Verification items for the finished model (mm, model axes). Give positions to 0.01 mm unless a question says otherwise; leave off trailing zeros. Loops run counter-clockwise (first coordinate to the right, second up) from the corner with the lowest first, then second, coordinate; pieces in that order, holes last. Notation, with made-up numbers: M 70.5,87.5 L 106.5,87.5 A32 cw 106.5,118.5 Z; hole C -1.5,53.5 d11. An arc over 180 degrees is marked long. Use CSV: the item, a comma, the result in double quotes.
from build123d import *

# Parameters (mm, degrees)
IZIM1_R                     = 3
Y_KSEKLIK_EKSTR_ZYON6_DEPTH = 99
IZIM2_R                     = 2
Y_KSEKLIK_EKSTR_ZYON7_DEPTH = 4
RADYUS1_SIZE                = 0.5
Y_KSEKLIK_EKSTR_ZYON8_START = 4
IZIM5_R                     = 2
Y_KSEKLIK_EKSTR_ZYON8_DEPTH = 4
RADYUS2_SIZE                = 0.5


with BuildPart() as part:
    # Çizim1 → Yükseklik-Ekstrüzyon6 (new, symmetric)
    with BuildSketch(Plane(origin=(0, 0, 0), x_dir=(1, 0, 0), z_dir=(0, 1, 0))):
        with Locations(Location((0, 0, 0), (0, 0, 270))):
            Circle(IZIM1_R)
    extrude(amount=Y_KSEKLIK_EKSTR_ZYON6_DEPTH, both=True)

    # Çizim2 → Yükseklik-Ekstrüzyon7 (add)
    with BuildSketch(Plane(origin=(0, 99, 0), x_dir=(1, 0, 0), z_dir=(0, 1, 0))):
        with Locations(Location((0, 0, 0), (0, 0, 270))):
            Circle(IZIM2_R)
    extrude(amount=Y_KSEKLIK_EKSTR_ZYON7_DEPTH)

    # Radyus1
    # a fillet whose section is not a circle: 0.5 mm, written as the material it takes off along each edge
    with BuildSketch(Plane(origin=(0, 103, 0), x_dir=(0, 0, 1), z_dir=(-1, 0, 0))) as radyus1_piece_1:
        with BuildLine():
            Bezier((2, -RADYUS1_SIZE), (2, 0), (2 - RADYUS1_SIZE, 0), weights=[1, 0.035355339, 1])
            Line((2 - RADYUS1_SIZE, 0), (2, 0))
            Line((2, 0), (2, -RADYUS1_SIZE))
        make_face()
    revolve(axis=Axis((0, 103, 0), (0, 1, 0)), mode=Mode.SUBTRACT)

    # Çizim5 → Yükseklik-Ekstrüzyon8 (add)
    with BuildSketch(Plane.XZ.offset(99).offset(Y_KSEKLIK_EKSTR_ZYON8_START)):
        with Locations(Location((0, 0, 0), (0, 0, 90))):
            Circle(IZIM5_R)
    extrude(amount=-Y_KSEKLIK_EKSTR_ZYON8_DEPTH)

    # Radyus2
    # a fillet whose section is not a circle: 0.5 mm, written as the material it takes off along each edge
    with BuildSketch(Plane(origin=(0, -103, 0), x_dir=(0, 0, 1), z_dir=(1, 0, 0))) as radyus2_piece_1:
        with BuildLine():
            Bezier((2, -RADYUS2_SIZE), (2, 0), (2 - RADYUS2_SIZE, 0), weights=[1, 0.035355339, 1])
            Line((2 - RADYUS2_SIZE, 0), (2, 0))
            Line((2, 0), (2, -RADYUS2_SIZE))
        make_face()
    revolve(axis=Axis((0, -103, 0), (0, -1, 0)), mode=Mode.SUBTRACT)


solid = part.part
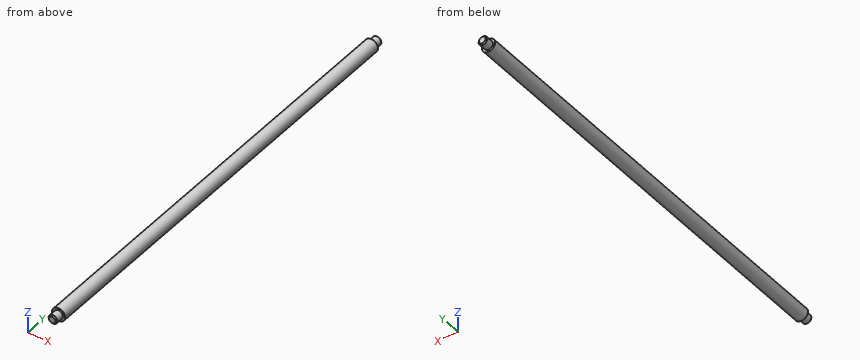
(1) Scan lines: L1, parallel to Z at x = 0.1, y = 55; L2, parallel to Y at x = 0.25, z = -2.7; L3, parallel to Z at x = 2.6, y = -38.5. Record each from-to range of solid material in increasing order. Write a range as from..to.
Calculated:
L1,"z = -3..3"
L2,"y = -99..99"
L3,"z = -1.5..1.5"
(2) Depth check by flat-ended pin: pin 1 Ø2 at (x, y) = (-1.5, -72.5) entering from +Z; pin 2 Ø3 at (x, z) = (1.5, -2) entering from +Y. Enter the tip coordinate at first touch or a pass-through.
Calculated:
pin 1,"stops at z = 2.96"
pin 2,"stops at y = 103"
(3) Section check A-A on y = -52. Record the cut outline in (x, z), plus the area to 3 significant figures.
Calculated:
outline,"C 0,0 d6"
area,"28.3 mm²"
